Check sheet for the modelled part. Datum: model origin and axes. Units: mm. A direction names the side the tool comes from. Give positions to 0.01 mm unless a question says otherwise; leave off trailing zeros. Write each loop counter-clockwise with the first axis right and the second up, starting at its lowest first coordinate (ties: lowest second). Pieces come first, ordered by that corner, then holes. Notation, with made-up numbers: (70.5, 15.25) -> (82.5, 15.25) arc R9 cw to (82.5, 28.25) -> close; hole circle Ø6 at (2.5, 11). An arc over 180 degrees is marked (long way). Answer as a JSON object with one key per item and string values.
from build123d import *

# Parameters (mm, degrees)
SKETCH1_W           = 73.66
SKETCH1_H           = 36.83
SKETCH1_R           = 1.0999978
SKETCH1_R_2         = 2.159
BOSS_EXTRUDE1_DEPTH = 40.64
SKETCH3_R           = 2.54
CUT_EXTRUDE2_DEPTH  = 38.1
SKETCH4_W           = 18.415
SKETCH4_H           = 36.83
CUT_EXTRUDE3_DEPTH  = 38.1


with BuildPart() as part:
    # Sketch1 → Boss-Extrude1 (new body)
    with BuildSketch(Plane(origin=(0, 0, 0), x_dir=(1, 0, 0), z_dir=(0, 1, 0))):
        with Locations((-1.422532637, -3.27613577)):
            Rectangle(SKETCH1_W, SKETCH1_H)
        with Locations(Location((-16.422528037, 11.72385963, 0), (0, 0, 270))):
            Circle(SKETCH1_R, mode=Mode.SUBTRACT)
        with Locations(Location((13.577462763, 11.72385963, 0), (0, 0, 90))):
            Circle(SKETCH1_R, mode=Mode.SUBTRACT)
        with Locations(Location((13.577462763, -18.27613117, 0), (0, 0, 270))):
            Circle(SKETCH1_R, mode=Mode.SUBTRACT)
        with Locations(Location((-16.422528037, -18.27613117, 0), (0, 0, 90))):
            Circle(SKETCH1_R, mode=Mode.SUBTRACT)
        with Locations(Location((31.597467363, -15.34113577, 0), (0, 0, 270))):
            Circle(SKETCH1_R_2, mode=Mode.SUBTRACT)
        with Locations(Location((31.597467363, 8.78886423, 0), (0, 0, 90))):
            Circle(SKETCH1_R_2, mode=Mode.SUBTRACT)
        with Locations(Location((-34.442532637, -15.34113577, 0), (0, 0, 90))):
            Circle(SKETCH1_R_2, mode=Mode.SUBTRACT)
        with Locations(Location((-34.442532637, 8.78886423, 0), (0, 0, 270))):
            Circle(SKETCH1_R_2, mode=Mode.SUBTRACT)
    extrude(amount=BOSS_EXTRUDE1_DEPTH)

    # Sketch3 → Cut-Extrude2 (cut)
    with BuildSketch(Plane.XZ):
        with Locations(Location((-16.422528037, 18.27613117, 0), (0, 0, 270))):
            Circle(SKETCH3_R)
        with Locations(Location((13.577462763, 18.27613117, 0), (0, 0, 270))):
            Circle(SKETCH3_R)
        with Locations(Location((13.577462763, -11.72385963, 0), (0, 0, 270))):
            Circle(SKETCH3_R)
        with Locations(Location((-16.422528037, -11.72385963, 0), (0, 0, 270))):
            Circle(SKETCH3_R)
    extrude(amount=-CUT_EXTRUDE2_DEPTH, mode=Mode.SUBTRACT)

    # Sketch4 → Cut-Extrude3 (cut)
    with BuildSketch(Plane(origin=(0, 40.64, 0), x_dir=(1, 0, 0), z_dir=(0, 1, 0))):
        with Locations((-29.045032637, -3.27613577)):
            Rectangle(SKETCH4_W, SKETCH4_H)
        with Locations((26.199967363, -3.27613577)):
            Rectangle(SKETCH4_W, SKETCH4_H)
    extrude(amount=-CUT_EXTRUDE3_DEPTH, mode=Mode.SUBTRACT)


solid = part.part
1. Access from +Z, -Z, +X, -X, +Y, -Y to the whole of each face (thin tool, end or side, straight path). Record for faces 4 (the face through (13, 38.1, 17)), 5 (the face through (16.992, 22, 4)), 6 (the face through (-29, 2.54, 3)).
Determined:
{"face 4": "-Y", "face 5": "+Z, -Z, +X, +Y", "face 6": "+Z, -Z, -X, +Y"}
2. Go/stop test with flat-tipped pins: P1, Ø18.5, axis at y = 18, z = -3.5, coming from the -X side; P2, Ø3.5, axis at x = 31.6, z = -8.79, coming from the +Y side; P3, Ø1.5, axis at x = 14, z = 19.5, coming from the -Y side; P4, Ø12, axis at y = 16, z = 18, coming from the +X side. Record where each tip stops, or that it passes through.
Determined:
{"P1": "x = -19.84", "P2": "through", "P3": "y = 38.1", "P4": "x = 16.99"}
3. Scan lines: L1, parallel to X at y = 34, z = 19.5; L2, parallel to Z at x = -14.5, y = 38; L3, parallel to X at y = 29.5, z = 16.5. Record each from-to range of solid material in increasing order. Write a range as [from, to].
Determined:
{"L1": "[-19.84, -18.65], [-14.2, 11.35], [15.8, 16.99]", "L2": "[-15.14, -13.38], [-10.06, 16.62], [19.94, 21.69]", "L3": "[-19.84, -18.24], [-14.61, 11.76], [15.39, 16.99]"}
4. Sectioned sample at A-A, the plane z = 4. Enter the section's corners in (x, y).
Determined:
{"outline": "(-38.25, 0) -> (35.41, 0) -> (35.41, 2.54) -> (16.99, 2.54) -> (16.99, 40.64) -> (-19.84, 40.64) -> (-19.84, 2.54) -> (-38.25, 2.54) -> close"}
5. Sectioned sample at B-B, the plane y = 34. Enter the section's corners in (x, z).
Determined:
{"outline": "(-19.84, -15.14) -> (16.99, -15.14) -> (16.99, 21.69) -> (-19.84, 21.69) -> close; hole circle Ø5.08 at (-16.42, -11.72); hole circle Ø5.08 at (-16.42, 18.28); hole circle Ø5.08 at (13.58, -11.72); hole circle Ø5.08 at (13.58, 18.28)"}
6. Mould release check, pull along Z, two halves, no side actions. Record for faces 1 (the face through (-2, 40.64, 3)), 2 (the face through (-2, 20, -15.139)), 3 (the face through (-15.753, 39.352, 19.149)): released by +Z, released by -Z, zero draft, split by the parting line, or undercut.
Determined:
{"face 1": "zero draft", "face 2": "released by -Z", "face 3": "undercut"}
